Model file for the job. Use its own axes, mm. Round coordinates to 2 decimals unless told otherwise and drop trailing zeros. Order: outer loops, then holes, each group sorted by start corner. A loop starts at its lowest first (then second) coordinate and runs counter-clockwise, first axis right, second up. Notation, with made-up numbers: (75, 83.5) - (95, 83.5) arc R24 cw to (95, 114.5) - close; hole circle Ø9 at (75.5, 6). An arc over 180 degrees is marked (long way). Use one line per item in the form item = value.
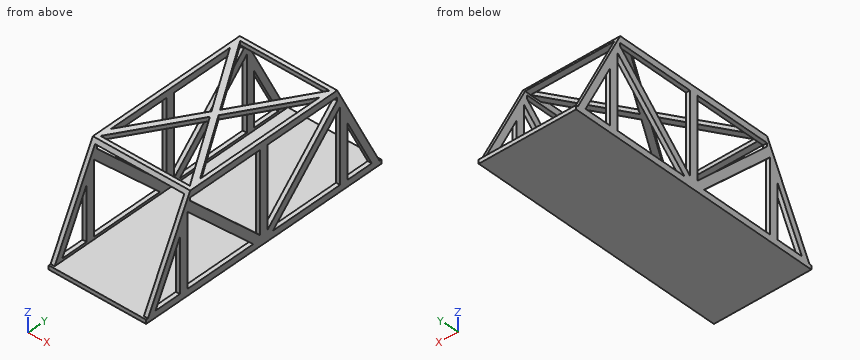
from build123d import *

# Parameters (mm, degrees)
F1_DEPTH = 38.1
F2_W     = 69.85
F2_H     = 69.85
F3_DEPTH = 127
F5_DEPTH = 76.2
F7_DEPTH = 5.588
F8_W     = 5.08
F8_H     = 3.175
F9_DEPTH = 76.2


with BuildPart() as f1:
    # F0 (on Right) → F1 (new body, symmetric)
    with BuildSketch(Plane.YZ):
        Polygon((-63.5, 32.0970378816), (-101.6, -44.1029621184), (101.6, -44.1029621184), (63.5, 32.0970378816), align=None)
    extrude(amount=F1_DEPTH, both=True)

    # F2 (on Front) → F3 (cut, symmetric)
    with BuildSketch(Plane.XZ):
        with Locations((0, -6.0029621184)):
            Rectangle(F2_W, F2_H)
    extrude(amount=F3_DEPTH, both=True, mode=Mode.SUBTRACT)

    # F4 (on face) → F5 (cut)
    with BuildSketch(Plane.YZ.offset(38.1)):
        Polygon((-72.39, 2.9578125559), (-93.3803873372, -39.0229621184), (-72.39, -39.0229621184), align=None)
        Polygon((-66.04, 18.0367817605), (-66.04, -39.0229621184), (-8.9802561211, -39.0229621184), align=None)
        Polygon((-3.175, 27.0170378816), (-63.5, 27.0170378816), (-63.5, 24.4770378816), (-3.175, -35.8479621184), align=None)
        Polygon((63.5, 27.0170378816), (3.175, 27.0170378816), (3.175, -35.8479621184), (63.5, 24.4770378816), align=None)
        Polygon((66.04, 18.5374412686), (8.0518, -39.0229621184), (66.04, -39.0229621184), align=None)
        Polygon((72.39, -39.0229621184), (93.3803873372, -39.0229621184), (72.39, 2.9578125559), align=None)
    extrude(amount=-F5_DEPTH, mode=Mode.SUBTRACT)

    # F6 (on face) → F7 (cut)
    with BuildSketch(Plane.XY.offset(32.0970378816)):
        Polygon((-34.925, 51.435), (-34.925, -51.435), (-2.778125, 0), align=None)
        Polygon((0, 4.445), (34.925, 60.325), (-34.925, 60.325), align=None)
        Polygon((2.778125, 0), (34.925, -51.435), (34.925, 51.435), align=None)
        Polygon((-34.925, -60.325), (34.925, -60.325), (0, -4.445), align=None)
    extrude(amount=-F7_DEPTH, mode=Mode.SUBTRACT)

    # F8 (on face) → F9 (join)
    with BuildSketch(Plane.YZ.offset(38.1)):
        with Locations((-99.06, -42.5154621184)):
            Rectangle(F8_W, F8_H)
        with Locations((99.06, -42.5154621184)):
            Rectangle(F8_W, F8_H)
    extrude(amount=-F9_DEPTH)


solid = f1.part
(1) Slice it at C-C on y = 80. Give the cut face in (x, z) (3 decimals), then the cut area to 3 significant figures.
Report:
outline = (-38.1, -44.103) - (38.1, -44.103) - (38.1, -39.023) - (34.925, -39.023) - (34.925, -40.928) - (-34.925, -40.928) - (-34.925, -39.023) - (-38.1, -39.023) - close; (-38.1, -12.262) - (-34.925, -12.262) - (-34.925, -0.903) - (-38.1, -0.903) - close; (34.925, -12.262) - (38.1, -12.262) - (38.1, -0.903) - (34.925, -0.903) - close
area = 326 mm2
(2) Slice it at B-B on y = -46.5. Count the separate pieces of the cut face and the enclosed holes in it, then the cut area to 3 significant figures.
Report:
separate_pieces = 7
enclosed_holes = 0
area = 379 mm2
(3) Probe probe 1 along X at (y, z) = (71, 7.5) (3 decimals); probe 2 along Z at (x, y) = (6.5, -71.5). List the from-to ranges inside material, lowest first. Write a range as [from, to].
Report:
probe_1 = [-38.1, -34.925], [34.925, 38.1]
probe_2 = [-44.1, -40.93]
(4) Slice it at A-A on x = -8. Give the cut face in (y, z) (1 decimal).
Report:
outline = (-101.6, -44.1) - (101.6, -44.1) - (101.6, -40.9) - (-101.6, -40.9) - close; (-65.1, 28.9) - (-60.3, 28.9) - (-60.3, 32.1) - (-63.5, 32.1) - close; (-17.2, 28.9) - (-8.4, 28.9) - (-8.4, 32.1) - (-17.2, 32.1) - close; (8.4, 28.9) - (17.2, 28.9) - (17.2, 32.1) - (8.4, 32.1) - close; (60.3, 28.9) - (65.1, 28.9) - (63.5, 32.1) - (60.3, 32.1) - close
(5) Pin check, flat tips, straight feed: pin 1 (1 mm diameter, centred on x = -36.5, z = -25.5, fed in from +Y); pin 2 (12 mm diameter, centred on y = -22.5, z = -36, fed in from +X); pin 3 (2.5 mm diameter, centred on x = 36.5, z = -11, fed in from +Y); pin 4 (2 mm diameter, centred on x = -37, z = 25.5, fed in from +Y). Stop position of each tip, or through.
Report:
pin_1 = 92.55
pin_2 = 38.1
pin_3 = 85.67
pin_4 = 67.3
